Autodesk Inventor part; units mm, degrees
sketch "Эскиз5" plane through (0, 0, 0) normal (0, 1, 0) x (-1, 0, 0)
  circle A0 centre (0, 0) radius 16.5
  dimension "d12" = 33
extrude "Выдавливание4" add sketch "Эскиз5" along normal blind 1
sketch "Эскиз7" plane through (0, 1, 0) normal (0, 1, 0) x (1, 0, 0)
  circle A0 centre (0, 0) radius 16
  circle A1 centre (0, 0) radius 16.5
  arc A2 (-0.5, 14.9917) -> (-0.5354, 14.9904) centre (0, 0) ccw
  line L0 (0.5, -14) -> (-0.5, -14)
  line L1 (-0.5, 14) -> (0.5, 14)
  line L2 (0.5, -14) -> (-0.5, 14) construction
  line L3 (-0.5, -14) -> (0.5, 14) construction
  line L4 (-0.5, -14) -> (0.5, -14)
  line L5 (0.5, -14) -> (0.5, -15.4866)
  line L6 (0.5, -15.4866) -> (-0.5, -15.4866)
  line L7 (-0.5, -15.4866) -> (-0.5, -14)
  line L8 (0.5, 14) -> (-0.5, 14)
  line L9 (-0.5, 14) -> (-0.5, 15.7701)
  line L10 (-0.5, 15.7701) -> (0.5, 15.7701)
  line L11 (0.5, 15.7701) -> (0.5, 14)
  arc A3 (0.5, -14.9917) -> (0.5354, 14.9904) centre (0, 0) ccw
  arc A4 (0.5354, 14.9904) -> (0.5, 14.9917) centre (0, 0) ccw
  arc A5 (-0.5354, 14.9904) -> (-0.5, -14.9917) centre (0, 0) ccw
  dimension "d17" = 1
  dimension "d18" = 28
  dimension "d19" = 32
  dimension "d21" = 2.045
  dimension "d22" = 177.955
  dimension "d23" = 0
  dimension "d24" = 1.7701
  dimension "d25" = 31.2568
  dimension "d26" = 0.5
  dimension "d27" = 15.7701
  dimension "d30" = 15
  dimension "d31" = 15
extrude "Выдавливание6" add sketch "Эскиз7" along normal blind 1 contours L9 L1 L11 A4 A3 L5 L0 L7 A5 A2
sketch "Эскиз9" plane through (0, 0, 0) normal (0, -1, 0) x (1, 0, 0)
  circle A0 centre (0, 0) radius 15
  circle A1 centre (0, 0) radius 14
  dimension "d41" = 30
  dimension "d42" = 28
extrude "Выдавливание8" add sketch "Эскиз9" along normal blind 10
properties part number "Крышка и батарейный отсек"
Part model, mm, in its own coordinate system. A direction names the side the tool comes from. Give positions to 0.01 mm unless a question says otherwise; leave off trailing zeros. Order: outer loops, then holes, each group sorted by start corner. A loop starts at its lowest first (then second) coordinate and runs counter-clockwise, first axis right, second up. Notation, with made-up numbers: M 46,66 L 86,66 A22 cw 86,77 Z; hole C 8,50 d1. An arc over 180 degrees is marked long. Use a Markdown table: item, result. Add a question column.
(1) Mould opens along X. For faces 5 (the face through (-14.985, -4.93, -0.66)), 6 (the face through (0.5, 1.5, 14.5)), 7 (the face through (0, 1.5, -14)), 8 (the face through (-14.996, 1.493, 0.34)) say: +X half, -X half, draft (parallel to the pull), parting line (faces both ways), or undercut.
(2) Saw through at B-B, the plane z = 0. Give the cut face in (x, y).
(3) Saw through at C-C, the plane y = -1.75. Give the cut face in (x, z), and give its area (3 significant figures).
(4) 3-axis set-ups, long thin cutter, end or side, ignore diameter. For faces 1 (the face through (0.5, 1.5, -14.5)), 2 (the face through (12.932, -4.93, 5.362)), 3 (the face through (0, 1.5, 14)), 4 (the face through (14.997, 1.493, -0.305)): which of +Z, -Z, +X, -X, +Y, -Y reach the whole face in a straight line?
(5) Probe line 1 along X through (y, z) = (-8.5, -0.5); line 2 along X through (y, z) = (-9.25, -6); line 3 along Z through (x, y) = (-5, -8.25). List the from-to ranges inside material, lowest first. Write a range as [from, to].
(6) Saw through at A-A, the plane x = 0. Give the cut face in (y, z), and give its area (3 significant figures).
(7) Drop flat-ended pins along their axis: P1, Ø4, axis at x = -8, z = 8.5, coming from the -Y side; P2, Ø0.5, axis at x = 0, y = 1.5, coming from the +Z side; P3, Ø1.5, axis at y = -7.5, z = -6, coming from the -X side. Give the stop position or say it passes through.
(8) Saw through at D-D, the plane y = 0.5. Give the cut face in (x, z), and give its area (3 significant figures).
Answer key:
| question | item | result |
|---|---|---|
| 1 | face 5 | parting line |
| 1 | face 6 | undercut |
| 1 | face 7 | undercut |
| 1 | face 8 | -X half |
| 2 | outline | M -16.5,0 L -15,0 L -15,-10 L -14,-10 L -14,0 L 14,0 L 14,-10 L 15,-10 L 15,0 L 16.5,0 L 16.5,1 L 15,1 L 15,2 L -15,2 L -15,1 L -16.5,1 Z |
| 3 | outline | C 0,0 d30; hole C 0,0 d28 |
| 3 | area | 91.1 mm^2 |
| 4 | face 1 | -Z, +Y |
| 4 | face 2 | -Y |
| 4 | face 3 | +Z, +Y |
| 4 | face 4 | +X, +Y |
| 5 | line 1 | [-14.99, -13.99], [13.99, 14.99] |
| 5 | line 2 | [-13.75, -12.65], [12.65, 13.75] |
| 5 | line 3 | [-14.14, -13.08], [13.08, 14.14] |
| 6 | outline | M -10,-15 L 0,-15 L 0,-16.5 L 1,-16.5 L 1,-14 L 2,-14 L 2,14 L 1,14 L 1,16.5 L 0,16.5 L 0,15 L -10,15 L -10,14 L 0,14 L 0,-14 L -10,-14 Z |
| 6 | area | 81.0 mm^2 |
| 7 | P1 | y = 0 |
| 7 | P2 | z = 14 |
| 7 | P3 | x = -14.05 |
| 8 | outline | C 0,0 d33 |
| 8 | area | 855 mm^2 |
